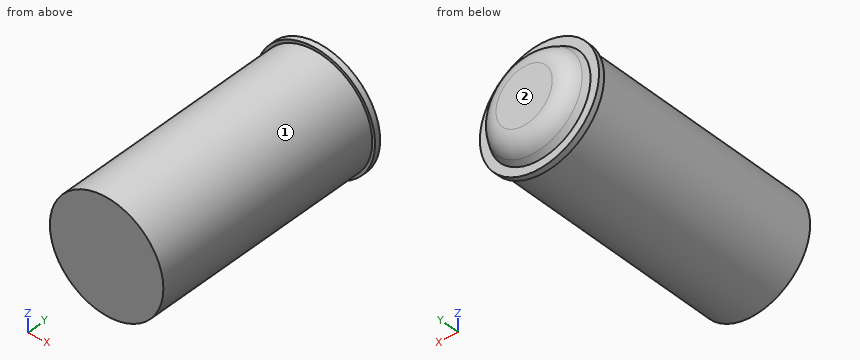
from build123d import *

# Parameters (mm, degrees)
SKETCH1_R           = 12.7
BOSS_EXTRUDE1_DEPTH = 1.27
SKETCH2_R           = 12.7
SKETCH2_R_2         = 11.43
SKETCH2_R_3         = 1.27
SKETCH2_R_4         = 2.54
BOSS_EXTRUDE2_DEPTH = 50.8
SKETCH3_R           = 13.335
BOSS_EXTRUDE3_DEPTH = 1.27
SKETCH4_R           = 11.43
BOSS_EXTRUDE4_DEPTH = 3.81
BOSS_EXTRUDE4_TAPER = 30
FILLET1_R           = 5.08


with BuildPart() as part:
    # Sketch1 → Boss-Extrude1 (new body)
    with BuildSketch(Plane(origin=(0, 0, 0), x_dir=(1, 0, 0), z_dir=(0, 1, 0))):
        Circle(SKETCH1_R)
    extrude(amount=BOSS_EXTRUDE1_DEPTH)

    # Sketch2 → Boss-Extrude2 (add)
    with BuildSketch(Plane(origin=(0, 1.27, 0), x_dir=(1, 0, 0), z_dir=(0, 1, 0))):
        Circle(SKETCH2_R)
        Circle(SKETCH2_R_2, mode=Mode.SUBTRACT)
        with Locations((-6.35, 0)):
            Circle(SKETCH2_R_3)
        with Locations((-4.490128061, 4.490128061)):
            Circle(SKETCH2_R_3)
        with Locations((-4.490128061, -4.490128061)):
            Circle(SKETCH2_R_3)
        Circle(SKETCH2_R_4)
        with Locations((0, 6.35)):
            Circle(SKETCH2_R_3)
        with Locations((4.490128061, 4.490128061)):
            Circle(SKETCH2_R_3)
        with Locations((6.35, 0)):
            Circle(SKETCH2_R_3)
        with Locations((4.490128061, -4.490128061)):
            Circle(SKETCH2_R_3)
        with Locations((0, -6.35)):
            Circle(SKETCH2_R_3)
    extrude(amount=BOSS_EXTRUDE2_DEPTH)

    # Sketch3 → Boss-Extrude3 (add)
    with BuildSketch(Plane(origin=(0, 52.07, 0), x_dir=(1, 0, 0), z_dir=(0, 1, 0))):
        Circle(SKETCH3_R)
    extrude(amount=BOSS_EXTRUDE3_DEPTH)

    # Sketch4 → Boss-Extrude4 (add)
    with BuildSketch(Plane(origin=(0, 53.34, 0), x_dir=(1, 0, 0), z_dir=(0, 1, 0))):
        Circle(SKETCH4_R)
    extrude(amount=BOSS_EXTRUDE4_DEPTH, taper=BOSS_EXTRUDE4_TAPER)

    # Fillet1
    fillet1_edges = [part.edges().sort_by_distance(p)[0] for p in [
        (-9.230295474, 57.15, 0),
    ]]
    fillet(fillet1_edges, radius=FILLET1_R)


solid = part.part
Could you check a few things on this model? Use its own coordinates, in mm. Face numbers are marked on the shaded views. A direction names the side the tool comes from. Coordinates: 2 decimals unless noted, no trailing zeros.
Q1. Please list where these lines run through material, in increasing order: L1, parallel to Z at x = 0, y = 30; L2, parallel to Z at x = -4, y = 39.
Q2. Suppose I cut it at A-A on y = 37. Give the number of separate pieces and of enclosed holes in the cut face, and give its area (3 significant figures).
Q3. Will these pins go through, and if not, where does the flat tip stop? pin 1 (6 mm diameter, centred on x = 0, z = 10, fed in from -Y); pin 2 (4 mm diameter, centred on y = 16, z = -6, fed in from -X); pin 3 (1 mm diameter, centred on y = 14, z = -10, fed in from +X); pin 4 (5 mm diameter, centred on x = 0, y = 23.5, fed in from +Z).
Q4. Which directions (+Z, -Z, +X, -X, +Y, -Y) give clear straight access to the entire face, cutting with the end or side of a thin tool? Please do the marked faces 1 and 2.
Answer:
1. L1: z = -12.7 to -11.43, -7.62 to -5.08, -2.54 to 2.54, 5.08 to 7.62, 11.43 to 12.7
1. L2: z = -12.05 to -10.71, -5.66 to -3.32, 3.32 to 5.66, 10.71 to 12.05
2. separate pieces: 10
2. enclosed holes: 1
2. area: 157 mm2
3. pin 1: stops at y = 0
3. pin 2: stops at x = -12.05
3. pin 3: stops at x = 8.43
3. pin 4: stops at z = 12.7
4. face 1: -Y
4. face 2: +Z, -Z, +X, -X, +Y
